The model under review builds one solid part; all positions refer to its coordinate system, in mm. Face numbers are marked on the shaded views. A direction names the side the tool comes from. Round coordinates to 2 decimals unless told otherwise and drop trailing zeros. Order: outer loops, then holes, each group sorted by start corner. A loop starts at its lowest first (then second) coordinate and runs counter-clockwise, first axis right, second up. Notation, with made-up numbers: M 80.25,-11.5 L 105.25,-11.5 A16 ccw 105.25,-7.5 Z; hole C 27,60.5 d3. An arc over 180 degrees is marked long. Answer as a JSON object with one key per item and string values. Group by question number.
1. Mouldability with a two-part tool opening along Z and no side actions: class the marked faces 1, 2 and 3 as released by +Z, released by -Z, zero draft, split by the parting line, or undercut.
2. To check wall thickness, follow probe 1 along X at (y, z) = (6, -6); probe 2 along Z at (x, y) = (13.25, 0); probe 3 along X at (y, z) = (-2, -2). State the ranges of each line that lie inside material, in increasing order. Write a range as [from, to].
3. Add section C-C on x = 9. State the section outline as (y, z) points.
4. Machinability: for the marked faces 4 and 5, which of the approach directions +Z, -Z, +X, -X, +Y, -Y give a long, thin tool a straight path to every point of the face, cutting with its end or side? Answer none if there is none.
5. Clearance check with flat-ended pins moving along their axes: P1, Ø5, axis at x = 7, z = -5.5, coming from the -Y side; P2, Ø6.5, axis at y = -2, z = -1.5, coming from the -X side; P3, Ø6, axis at x = 11.5, y = -11, coming from the +Z side. State where each tip first meets the part, or that it passes through.
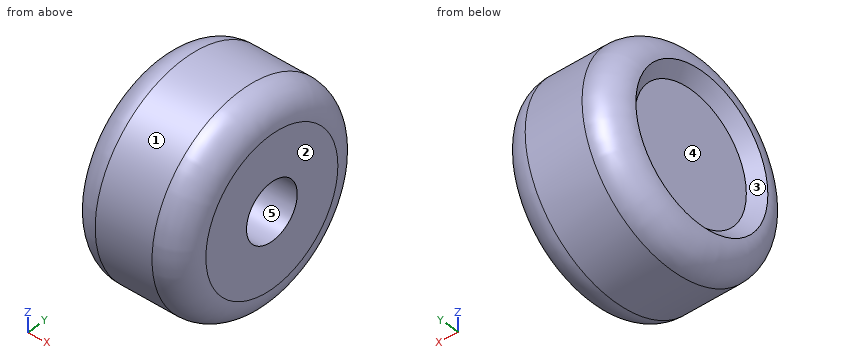
```python
from build123d import *

# Parameters (mm, degrees)
F0_R     = 18
F1_DEPTH = 20
F2_R     = 5
F3_DEPTH = 15
F4_R     = 5
F5_R     = 13
F6_DEPTH = 2
F7_SIZE  = 1.99999


# Not quite as in the source:
# - a fillet or chamfer is up to 0.001 mm smaller than in the source, because OpenCascade refuses the exact size


with BuildPart() as f1:
    # F0 (on Right) → F1 (new body)
    with BuildSketch(Plane.YZ):
        Circle(F0_R)
    extrude(amount=F1_DEPTH)

    # F2 (on face) → F3 (cut)
    with BuildSketch(Plane.YZ.offset(20)):
        Circle(F2_R)
    extrude(amount=-F3_DEPTH, mode=Mode.SUBTRACT)

    # F4
    f4_edges = [f1.edges().sort_by_distance(p)[0] for p in [
        (0, -18, 0),
        (20, -18, 0),
    ]]
    fillet(f4_edges, radius=F4_R)

    # F5 (on face) → F6 (cut)
    with BuildSketch(Plane(origin=(0, 0, 0), x_dir=(0, -1, 0), z_dir=(-1, 0, 0))):
        Circle(F5_R)
    extrude(amount=-F6_DEPTH, mode=Mode.SUBTRACT)

    # F7 (size 2 in the source; OpenCascade refuses exactly that, so slightly less here)
    f7_edges = [f1.edges().sort_by_distance(p)[0] for p in [
        (2, 13, 0),
    ]]
    chamfer(f7_edges, length=F7_SIZE)


solid = f1.part
```
Recorded:
{
 "1": {"face 1": "split by the parting line", "face 2": "zero draft", "face 3": "undercut"},
 "2": {"probe 1": "x = [2, 20]", "probe 2": "z = [-18, -5], [5, 18]", "probe 3": "x = [2, 5]"},
 "3": {"outline": "C 0,0 d36; hole C 0,0 d10"},
 "4": {"face 4": "-X", "face 5": "+X"},
 "5": {"P1": "stops at y = -17.75", "P2": "stops at x = 2", "P3": "stops at z = 16.12"}
}
